For this review, take the finished solid that the model builds, in its own axes (mm). A direction names the side the tool comes from. Give positions to 0.01 mm unless a question says otherwise; leave off trailing zeros. Write each loop counter-clockwise with the first axis right and the second up, starting at its lowest first coordinate (ties: lowest second). Pieces come first, ordered by that corner, then holes.
1) For P1, Ø3, axis at x = 0.5, y = 0.5, coming from the -Z side; P2, Ø2, axis at x = -3, z = -23.5, coming from the +Y side, all flat-tipped, find the tip position at first contact; note any pin that passes through.
2) We need section C-C on y = 0. Give the boundary of the cut face in (x, z).
3) Draft analysis for pull direction X (two halves, no side actions). For faces 6 (the face through (0.1, 4, -28.5)), 7 (the face through (5, 0, 3)), 8 (the face through (3, 0, -12)), 9 (the face through (-4.01, 0.33, 8.48)), state which applies: pulls with the +X half, pulls with the -X half, needs draft (parallel to the pull), parting line crosses it, or undercut.
4) We need section A-A on y = -4. Give the boundary of the cut face in (x, z), and give its area (3 significant figures).
5) Wall thickness on line 1 along Z through (x, y) = (4.35, 0); line 2 along Z through (x, y) = (-3.5, -3.75); line 3 along X through (y, z) = (-3.75, -31): over which ranges is each line inside the solid? List them lowest first.
6) Machinability: for faces 1 (the face through (0, -5, -28)), 2 (the face through (0, 0, -27)), 3 (the face through (-2.2, 2.3, -25)), 4 (the face through (0, 0, 2)), 5 (the face through (0.1, -4, -28.5)), which of the approach directions +Z, -Z, +X, -X, +Y, -Y give a long, thin tool a straight path to every point of the face, cutting with its end or side? Answer none if there is none.
7) We need section D-D on x = 2. Give the boundary of the cut face in (y, z).
8) We need section B-B on z = -31. Give the boundary of the cut face in (x, y), and give its area (3 significant figures).
from build123d import *

# Parameters (mm, degrees)
SKETCH1_W           = 10
SKETCH1_H           = 10
BOSS_EXTRUDE1_DEPTH = 2
SKETCH2_W           = 2
SKETCH2_H           = 10
BOSS_EXTRUDE2_DEPTH = 8
SKETCH3_R           = 2.5
CUT_EXTRUDE1_DEPTH  = 16
SKETCH4_R           = 3
BOSS_EXTRUDE3_DEPTH = 25
SKETCH5_W           = 10
SKETCH5_H           = 10
BOSS_EXTRUDE4_DEPTH = 2
SKETCH6_W           = 10
SKETCH6_H           = 2
BOSS_EXTRUDE5_DEPTH = 8
SKETCH7_R           = 2.5
CUT_EXTRUDE2_DEPTH  = 37.742346142


with BuildPart() as part:
    # Sketch1 → Boss-Extrude1 (new body)
    with BuildSketch(Plane.XY):
        Rectangle(SKETCH1_W, SKETCH1_H)
    extrude(amount=BOSS_EXTRUDE1_DEPTH)

    # Sketch2 → Boss-Extrude2 (add)
    with BuildSketch(Plane.XY.offset(2)):
        with Locations((-4, 0)):
            Rectangle(SKETCH2_W, SKETCH2_H)
        with Locations((4, 0)):
            Rectangle(SKETCH2_W, SKETCH2_H)
    extrude(amount=BOSS_EXTRUDE2_DEPTH)

    # Sketch3 → Cut-Extrude1 (cut, through all)
    with BuildSketch(Plane.ZY.offset(5)):
        with Locations(Location((6, 0, 0), (0, 0, 270))):
            Circle(SKETCH3_R)
    extrude(amount=-CUT_EXTRUDE1_DEPTH, mode=Mode.SUBTRACT)

    # Sketch4 → Boss-Extrude3 (add)
    with BuildSketch(Plane(origin=(0, 0, 0), x_dir=(-1, 0, 0), z_dir=(0, 0, -1))):
        Circle(SKETCH4_R)
    extrude(amount=BOSS_EXTRUDE3_DEPTH)

    # Sketch5 → Boss-Extrude4 (add)
    with BuildSketch(Plane(origin=(0, 0, -25), x_dir=(-1, 0, 0), z_dir=(0, 0, -1))):
        Rectangle(SKETCH5_W, SKETCH5_H)
    extrude(amount=BOSS_EXTRUDE4_DEPTH)

    # Sketch6 → Boss-Extrude5 (add)
    with BuildSketch(Plane(origin=(0, 0, -27), x_dir=(-1, 0, 0), z_dir=(0, 0, -1))):
        with Locations((0, -4)):
            Rectangle(SKETCH6_W, SKETCH6_H)
        with Locations((0, 4)):
            Rectangle(SKETCH6_W, SKETCH6_H)
    extrude(amount=BOSS_EXTRUDE5_DEPTH)

    # Sketch7 → Cut-Extrude2 (cut, through all)
    with BuildSketch(Plane.XZ.offset(5)):
        with Locations(Location((0, -31, 0), (0, 0, 270))):
            Circle(SKETCH7_R)
    extrude(amount=-CUT_EXTRUDE2_DEPTH, mode=Mode.SUBTRACT)


solid = part.part
Results list:
1. P1: stops at z = -27
1. P2: stops at y = 2.24
2. outline: (-5, -27) - (5, -27) - (5, -25) - (3, -25) - (3, 0) - (5, 0) - (5, 3.5) - (3, 3.5) - (3, 2) - (-3, 2) - (-3, 3.5) - (-5, 3.5) - (-5, 0) - (-3, 0) - (-3, -25) - (-5, -25) - close; (-5, 8.5) - (-3, 8.5) - (-3, 10) - (-5, 10) - close; (3, 8.5) - (5, 8.5) - (5, 10) - (3, 10) - close
3. face 6: undercut
3. face 7: pulls with the +X half
3. face 8: parting line crosses it
3. face 9: needs draft
4. outline: (-5, -35) - (5, -35) - (5, -25) - (-5, -25) - close; (-5, 0) - (5, 0) - (5, 10) - (3, 10) - (3, 2) - (-3, 2) - (-3, 10) - (-5, 10) - close; hole circle Ø5 at (0, -31)
4. area: 132 mm2
5. line 1: z = -27 to -25, 0 to 3.5, 8.5 to 10
5. line 2: z = -35 to -25, 0 to 10
5. line 3: x = -5 to -2.5, 2.5 to 5
6. face 1: +Z, -Z, +X, -X, -Y
6. face 2: -Z, +X, -X
6. face 3: none
6. face 4: +Z, +Y, -Y
6. face 5: +Y, -Y
7. outline: (-5, -35) - (-3, -35) - (-3, -32.5) - (-5, -32.5) - close; (-5, -29.5) - (-3, -29.5) - (-3, -27) - (3, -27) - (3, -29.5) - (5, -29.5) - (5, -25) - (2.24, -25) - (2.24, 0) - (5, 0) - (5, 2) - (-5, 2) - (-5, 0) - (-2.24, 0) - (-2.24, -25) - (-5, -25) - close; (3, -35) - (5, -35) - (5, -32.5) - (3, -32.5) - close
8. outline: (-5, -5) - (-2.5, -5) - (-2.5, -3) - (-5, -3) - close; (-5, 3) - (-2.5, 3) - (-2.5, 5) - (-5, 5) - close; (2.5, -5) - (5, -5) - (5, -3) - (2.5, -3) - close; (2.5, 3) - (5, 3) - (5, 5) - (2.5, 5) - close
8. area: 20.0 mm2
